Could you check a few things on this model? Use its own coordinates, in mm. Face numbers are marked on the shaded views. Round coordinates to 2 decimals unless told otherwise and drop trailing zeros. Loops run counter-clockwise (first coordinate to the right, second up) from the corner with the lowest first, then second, coordinate; pieces in that order, holes last. Notation, with made-up numbers: (36.25, 19.25) -> (50.25, 19.25) arc R20 ccw to (50.25, 39.25) -> close; hole circle Ø10 at (-23, -3.75). An arc over 180 degrees is marked (long way). One line per item, written item: value.
from build123d import *

# Parameters (mm, degrees)
SKETCH1_W           = 29.88277087
SKETCH1_H           = 5.669626998
SKETCH1_R           = 2
BOSS_EXTRUDE1_DEPTH = 2


with BuildPart() as part:
    # Sketch1 → Boss-Extrude1 (new body)
    with BuildSketch(Plane(origin=(0, 0, 0), x_dir=(0, 0, -1), z_dir=(1, 0, 0))):
        Rectangle(SKETCH1_W, SKETCH1_H)
        with Locations((-12, 0)):
            Circle(SKETCH1_R, mode=Mode.SUBTRACT)
        with Locations(Location((12, 0, 0), (0, 0, 180))):
            Circle(SKETCH1_R, mode=Mode.SUBTRACT)
    extrude(amount=BOSS_EXTRUDE1_DEPTH)


solid = part.part
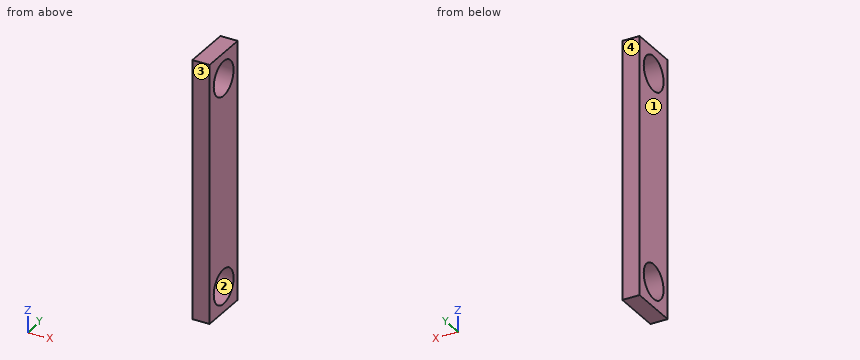
(1) I'm going to push a flat-ended pin straight in: pin 1 Ø3 at (y, z) = (0, -12) entering from -X. Where does the tip first touch, or does it pass through?
Recorded:
pin 1: through
(2) Thinking about a two-plate mould opening in Y: for the marked faces 1, 2, 3 and 4, which applies, released by +Y, released by -Y, zero draft, split by the parting line, or undercut?
Recorded:
face 1: zero draft
face 2: undercut
face 3: released by -Y
face 4: released by +Y
(3) If we section it at B-B, the plane z = -12: Please give me the cut outline in (x, y), then the cut area to 3 significant figures.
Recorded:
outline: (0, -2.83) -> (2, -2.83) -> (2, -2) -> (0, -2) -> close; (0, 2) -> (2, 2) -> (2, 2.83) -> (0, 2.83) -> close
area: 3.34 mm²
(4) If I drill on L1, parallel to Z at x = 1.1, y = 0.5; L2, parallel to Y at x = 0.65, z = -12; L3, parallel to Z at x = 1.45, y = 1.55, over which ranges is the centre line in solid material (lowest first)?
Recorded:
L1: -14.94 to -13.94, -10.06 to 10.06, 13.94 to 14.94
L2: -2.83 to -2, 2 to 2.83
L3: -14.94 to -13.26, -10.74 to 10.74, 13.26 to 14.94
(5) If we section it at C-C, the plane x = 0.95: Please give me the cut outline in (y, z).
Recorded:
outline: (-2.83, -14.94) -> (2.83, -14.94) -> (2.83, 14.94) -> (-2.83, 14.94) -> close; hole circle Ø4 at (0, -12); hole circle Ø4 at (0, 12)
(6) If we section it at D-D, the plane y = -1.75: Please give me the cut outline in (x, z).
Recorded:
outline: (0, -14.94) -> (2, -14.94) -> (2, -12.97) -> (0, -12.97) -> close; (0, -11.03) -> (2, -11.03) -> (2, 11.03) -> (0, 11.03) -> close; (0, 12.97) -> (2, 12.97) -> (2, 14.94) -> (0, 14.94) -> close
(7) If we section it at A-A, the plane y = 0: Please give me the cut outline in (x, z).
Recorded:
outline: (0, -14.94) -> (2, -14.94) -> (2, -14) -> (0, -14) -> close; (0, -10) -> (2, -10) -> (2, 10) -> (0, 10) -> close; (0, 14) -> (2, 14) -> (2, 14.94) -> (0, 14.94) -> close
